```python
from build123d import *

# Parameters (mm, degrees)
SKETCH1_R           = 1
SKETCH1_W           = 2.5
SKETCH1_H           = 2
BOSS_EXTRUDE4_DEPTH = 2


with BuildPart() as part:
    # Sketch1 → Boss-Extrude4 (new body)
    with BuildSketch(Plane(origin=(0, 0, 0), x_dir=(1, 0, 0), z_dir=(0, 1, 0))):
        with BuildLine():
            Line((4.461504525, -1.55), (10, -1.55))
            Line((10, -1.55), (10, -2))
            ThreePointArc((10, -2), (10.292893219, -2.707106781), (11, -3))
            Line((11, -3), (14.538495475, -3))
            ThreePointArc((14.538495475, -3), (15.245602257, -2.707106781), (15.538495475, -2))
            Line((15.538495475, -2), (15.538495475, 2))
            ThreePointArc((15.538495475, 2), (15.245602257, 2.707106781), (14.538495475, 3))
            Line((14.538495475, 3), (11, 3))
            ThreePointArc((11, 3), (10.292893219, 2.707106781), (10, 2))
            Line((10, 2), (10, 1.55))
            Line((10, 1.55), (4.461504525, 1.55))
            ThreePointArc((4.461504525, 1.55), (0, 0), (4.461504525, -1.55))
        make_face()
        with Locations((2.5, 0)):
            Circle(SKETCH1_R, mode=Mode.SUBTRACT)
        with Locations((13.839657546, 0)):
            Rectangle(SKETCH1_W, SKETCH1_H, mode=Mode.SUBTRACT)
    extrude(amount=BOSS_EXTRUDE4_DEPTH)


solid = part.part
```
Geometry check sheet. Reference: the model listing, model coordinates, mm. A direction names the side the tool comes from. Coordinates: 2 decimals unless noted, no trailing zeros. Write each loop counter-clockwise with the first axis right and the second up, starting at its lowest first coordinate (ties: lowest second). Pieces come first, ordered by that corner, then holes. Notation, with made-up numbers: M -31.5,-0.75 L 20.5,-0.75 A13 cw 20.5,16.25 Z; hole C 62,67.25 d5. An arc over 180 degrees is marked long. Answer as a JSON object with one key per item and string values.
1. Section check C-C, the plane y = 0.3. Enter the section's corners in (x, z), plus the area to 3 significant figures.
Answers below:
{"outline": "M 4.46,-1.55 L 10,-1.55 L 10,-2 A1 ccw 11,-3 L 14.54,-3 A1 ccw 15.54,-2 L 15.54,2 A1 ccw 14.54,3 L 11,3 A1 ccw 10,2 L 10,1.55 L 4.46,1.55 A2.5 ccw long Z; hole C 2.5,0 d2; hole M 12.59,-1 L 15.09,-1 L 15.09,1 L 12.59,1 Z", "area": "59.9 mm²"}
2. Draft check along X on faces 1 (the cylindrical face through (10.285, 0.986, 2.699)), 2 (the flat face through (13, 1, 3)), 3 (the flat face through (15.538, 1, 0)). Enter one of: released by +X, released by -X, zero draft, split by the parting line, or undercut.
Answers below:
{"face 1": "undercut", "face 2": "zero draft", "face 3": "released by +X"}
3. Scan lines: L1, parallel to X at y = 1.55, z = 0; L2, parallel to Z at x = 2.5, y = 0.65; L3, parallel to Z at x = 14, y = 0.45. Record each from-to range of solid material in increasing order.
Answers below:
{"L1": "x = 0 to 1.5, 3.5 to 12.59, 15.09 to 15.54", "L2": "z = -2.5 to -1, 1 to 2.5", "L3": "z = -3 to -1, 1 to 3"}
4. Section check B-B, the plane z = 0.55. Enter the section's corners in (x, y), plus the area to 3 significant figures.
Answers below:
{"outline": "M 0.06,0 L 1.66,0 L 1.66,2 L 0.06,2 Z; M 3.34,0 L 12.59,0 L 12.59,2 L 3.34,2 Z; M 15.09,0 L 15.54,0 L 15.54,2 L 15.09,2 Z", "area": "22.6 mm²"}
5. Tool access check on faces 4 (the cylindrical face through (10.301, 0.986, -2.715)), 5 (the flat face through (14, 1, -1)), 6 (the flat face through (7, 1, 1.55)), 7 (the cylindrical face through (15.25, 0.99, -2.7)). Record the directions out of +Z, -Z, +X, -X, +Y, -Y that give a thin tool (end or side, any length) a straight path to the whole face; none if there is none.
Answers below:
{"face 4": "-Z, +Y, -Y", "face 5": "+Y, -Y", "face 6": "+Z, +Y, -Y", "face 7": "-Z, +X, +Y, -Y"}
6. Section check D-D, the plane x = 9.25. Enter the section's corners in (y, z), plus the area to 3 significant figures.
Answers below:
{"outline": "M 0,-1.55 L 2,-1.55 L 2,1.55 L 0,1.55 Z", "area": "6.20 mm²"}
7. Section check A-A, the plane x = 2.5. Enter the section's corners in (y, z).
Answers below:
{"outline": "M 0,-2.5 L 2,-2.5 L 2,-1 L 0,-1 Z; M 0,1 L 2,1 L 2,2.5 L 0,2.5 Z"}
8. Go/stop test with flat-tipped pins: pin 1 Ø3 at (x, z) = (4, -1.5) entering from -Y; pin 2 Ø1.2 at (x, z) = (2.5, 0) entering from -Y. Record where each tip stops, or that it passes through.
Answers below:
{"pin 1": "stops at y = 0", "pin 2": "passes through"}
